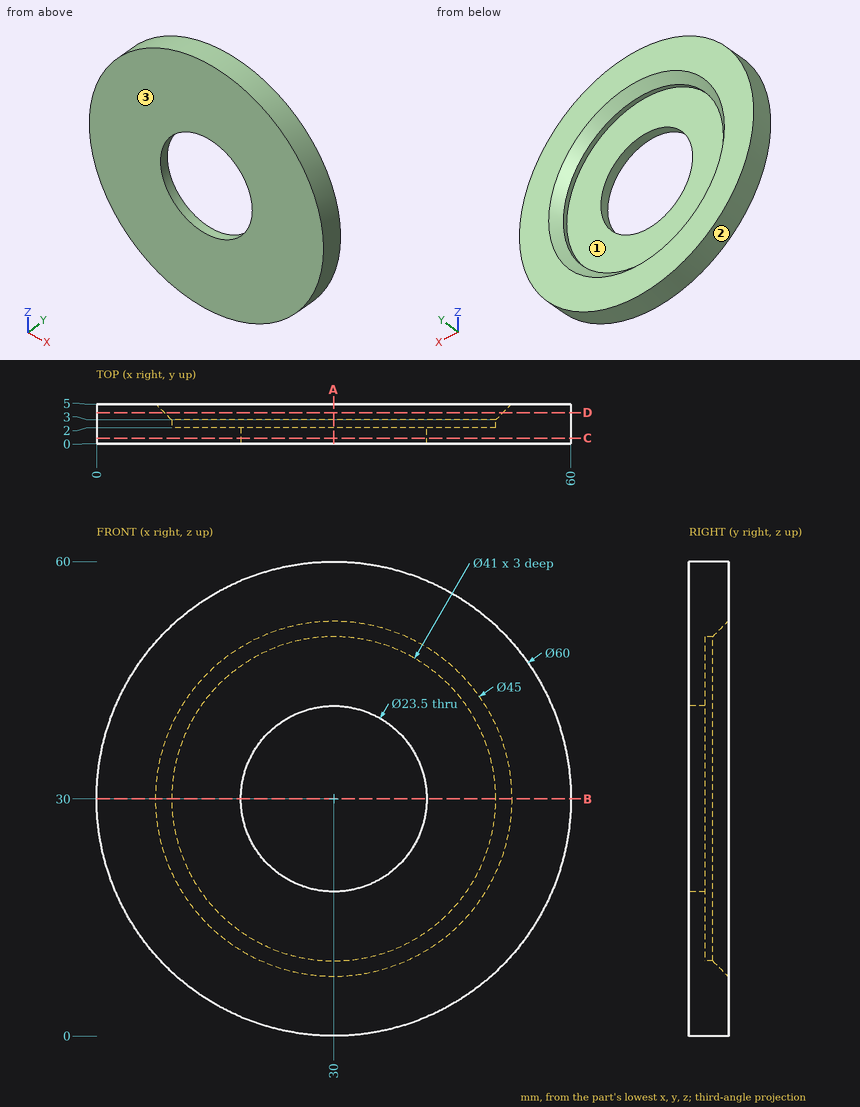
Drawing for the job (mm, zero at the part's lowest x, y, z). Round coordinates to 2 decimals unless told otherwise and drop trailing zeros. Write each loop counter-clockwise with the first axis right and the second up, starting at its lowest first coordinate (ties: lowest second). Pieces come first, ordered by that corner, then holes. Notation, with made-up numbers: M -36.75,86 L 2.25,86 A9 cw 2.25,99 Z; hole C -39.5,-36.5 d6. An arc over 180 degrees is marked long. Answer in a Markdown table with one row per item.
1. Saw through at A-A (x = 30). List the corners of the cut face in (y, z).
Geometry check:
| item | result |
|---|---|
| outline | M 0,0 L 5,0 L 5,7.5 L 3,9.5 L 2,9.5 L 2,18.25 L 0,18.25 Z; M 0,41.75 L 2,41.75 L 2,50.5 L 3,50.5 L 5,52.5 L 5,60 L 0,60 Z |
2. Saw through at C-C (y = 0.7). List the corners of the cut face in (x, z), and give its area (3 significant figures).
Geometry check:
| item | result |
|---|---|
| outline | C 30,30 d60; hole C 30,30 d23.5 |
| area | 2,390 mm2 |
3. Probe L1, parallel to Z at x = 30, y = 1.3; L2, parallel to Z at x = 30, y = 2.3; L3, parallel to Y at x = 48.5, z = 25. List the from-to ranges inside material, lowest first. Write a range as [from, to].
Geometry check:
| item | result |
|---|---|
| L1 | [0, 18.25], [41.75, 60] |
| L2 | [0, 9.5], [50.5, 60] |
| L3 | [0, 2] |
4. Saw through at D-D (y = 3.9). List the corners of the cut face in (x, z), and give its area (3 significant figures).
Geometry check:
| item | result |
|---|---|
| outline | C 30,30 d60; hole C 30,30 d42.8 |
| area | 1,390 mm2 |
5. Mould opens along X. For the marked faces 1, 2 and 3 say: +X half, -X half, draft (parallel to the pull), parting line (faces both ways), or undercut.
Geometry check:
| item | result |
|---|---|
| face 1 | undercut |
| face 2 | parting line |
| face 3 | draft |
6. Saw through at B-B (z = 30). List the corners of the cut face in (x, y), and give its area (3 significant figures).
Geometry check:
| item | result |
|---|---|
| outline | M 0,0 L 18.25,0 L 18.25,2 L 9.5,2 L 9.5,3 L 7.5,5 L 0,5 Z; M 41.75,0 L 60,0 L 60,5 L 52.5,5 L 50.5,3 L 50.5,2 L 41.75,2 Z |
| area | 126 mm2 |
7. Flat gauge pins, fed straight in: P1, Ø1.5, axis at y = 0.5, z = 20.5, coming from the +X side; P2, Ø8, axis at x = 11.5, z = 41, coming from the +Y side; P3, Ø3, axis at x = 33, y = 4, coming from the +Z side; P4, Ø3, axis at x = 15, z = 42, coming from the +Y side. Where does each tip first touch, or does it go through?
Geometry check:
| item | result |
|---|---|
| P1 | x = 58.7 |
| P2 | y = 5 |
| P3 | z = 59.96 |
| P4 | y = 3.21 |
